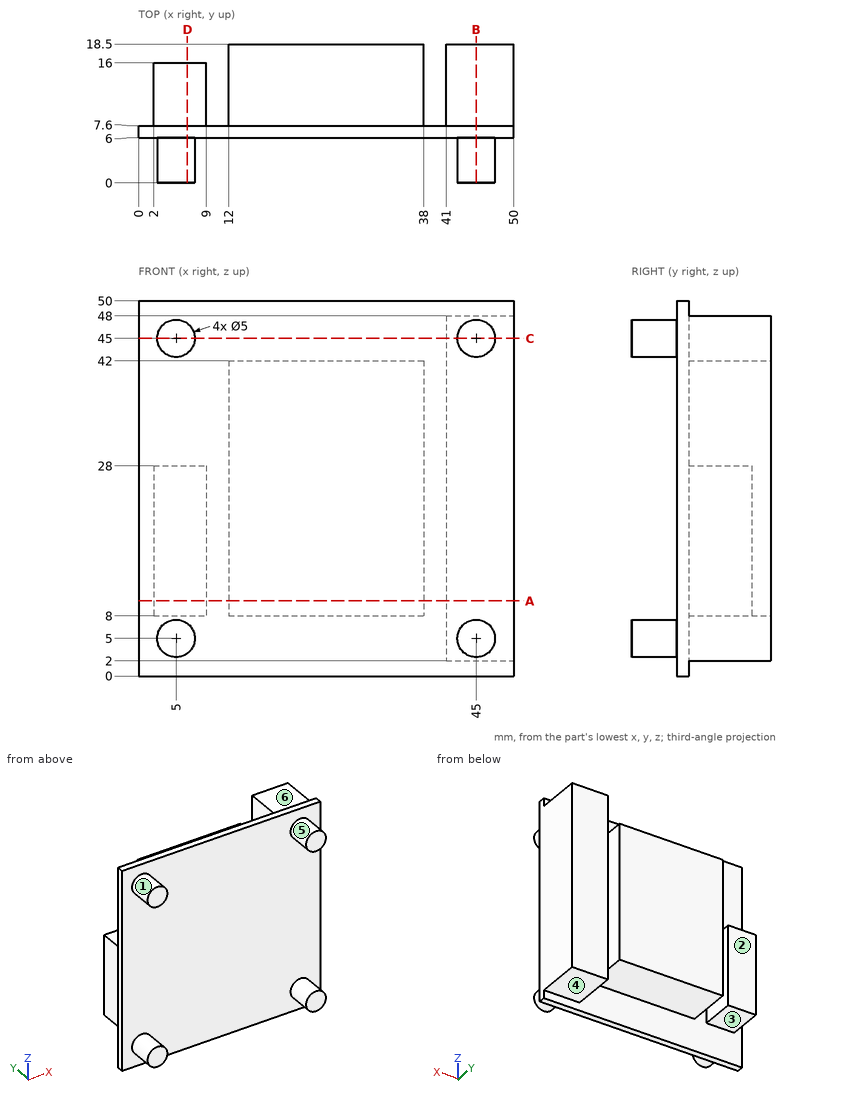
Study the drawing (mm; zero at the part's minimum x, y, z) and answer. A direction names the side the tool comes from. Give positions to 0.01 mm unless a question says otherwise; leave off trailing zeros. Loops run counter-clockwise (first coordinate to the right, second up) from the corner with the lowest first, then second, coordinate; pieces in that order, holes last. Notation, with made-up numbers: (63, -21.75) - (121, -21.75) arc R31 cw to (121, 7.25) - close; hole circle Ø8 at (-32.5, 55.25). An arc over 180 degrees is marked (long way). Answer as CSV lines item,"result". Start each with the question number.
1) Find section D-D (x = 6.5). Write down the section's boundary in (y, z), then the cut area to 3 significant figures.
2) Each of these flat-tipped pins is pushed along its axis until it touches: pin 1 Ø1.5 at (x, z) = (26.5, 26) entering from -Y; pin 2 Ø7.5 at (x, y) = (4.5, 12) entering from +Z; pin 3 Ø5.5 at (y, z) = (11.5, 22) entering from -X; pin 4 Ø3 at (y, z) = (3.5, 34) entering from +X. Where does it stop, or does it pass through?
3) Determine the mould class of the marked faces 1, 2 and 3 for opening direction Z: released by +Z, released by -Z, zero draft, split by the parting line, or undercut.
4) Which of the six approach directions +Z, -Z, +X, -X, +Y, -Y give full straight-line access (tool end or side, diameter ignored) to the marked faces 4, 5 and 6?
5) Find section B-B (x = 45). Write down the section's boundary in (y, z).
6) Find section A-A (z = 10). Write down the section's boundary in (x, y), then the cut area to 3 significant figures.
7) Find section C-C (z = 45). Write down the section's boundary in (x, y), then the cut area to 3 significant figures.
8) Straight lines are drawn through the part: L1, parallel to X at y = 14.5, z = 21; L2, parallel to X at y = 11, z = 36.5; L3, parallel to X at y = 11.5, z = 45.5. For each, find the intervals that lie inside material, in ascending order. Write a range as from..to.
Findings below:
1,outline,"(0, 3) - (6, 3) - (6, 0) - (7.6, 0) - (7.6, 8) - (16, 8) - (16, 28) - (7.6, 28) - (7.6, 50) - (6, 50) - (6, 47) - (0, 47) - (0, 43) - (6, 43) - (6, 7) - (0, 7) - close"
1,area,"296 mm^2"
2,pin 1,"y = 6"
2,pin 2,"z = 28"
2,pin 3,"x = 2"
2,pin 4,"through"
3,face 1,"undercut"
3,face 2,"zero draft"
3,face 3,"released by -Z"
4,face 4,"-Z, +X, -X, +Y"
4,face 5,"-Y"
4,face 6,"+Z, +X, -X, +Y"
5,outline,"(0, 2.5) - (6, 2.5) - (6, 0) - (7.6, 0) - (7.6, 2) - (18.5, 2) - (18.5, 48) - (7.6, 48) - (7.6, 50) - (6, 50) - (6, 47.5) - (0, 47.5) - (0, 42.5) - (6, 42.5) - (6, 7.5) - (0, 7.5) - close"
6,outline,"(0, 6) - (50, 6) - (50, 18.5) - (41, 18.5) - (41, 7.6) - (38, 7.6) - (38, 18.5) - (12, 18.5) - (12, 7.6) - (9, 7.6) - (9, 16) - (2, 16) - (2, 7.6) - (0, 7.6) - close"
6,area,"520 mm^2"
7,outline,"(0, 6) - (2.5, 6) - (2.5, 0) - (7.5, 0) - (7.5, 6) - (42.5, 6) - (42.5, 0) - (47.5, 0) - (47.5, 6) - (50, 6) - (50, 18.5) - (41, 18.5) - (41, 7.6) - (0, 7.6) - close"
7,area,"238 mm^2"
8,L1,"2..9, 12..38, 41..50"
8,L2,"12..38, 41..50"
8,L3,"41..50"
